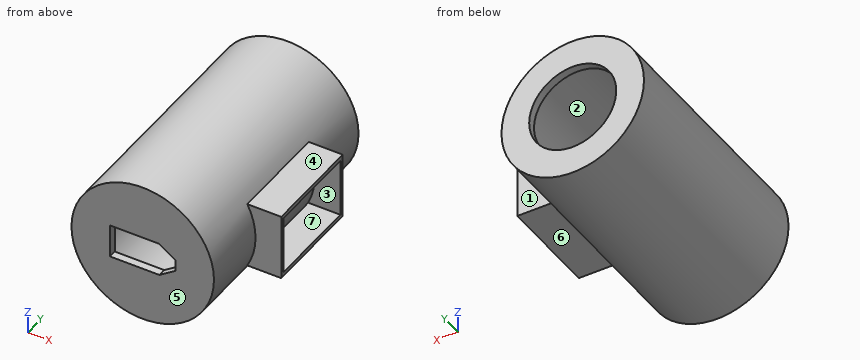
from build123d import *

# Parameters (mm, degrees)
F0_R     = 18
F0_R_2   = 16
F1_DEPTH = 60
F0_R_3   = 11
F2_DEPTH = 8
F3_W     = 25.5
F3_H     = 16.8
F3_W_2   = 23.5
F3_H_2   = 14.8
F4_DEPTH = 24.5
F5_DEPTH = 28.5
F6_DEPTH = 60
F7_DEPTH = 58
F8_DEPTH = 2


with BuildPart() as f1:
    # F0 (on Front) → F1 (new body)
    with BuildSketch(Plane.XZ):
        Circle(F0_R)
        Circle(F0_R_2, mode=Mode.SUBTRACT)
    extrude(amount=F1_DEPTH)

    # F0 (on Front) → F2 (join)
    with BuildSketch(Plane.XZ):
        Circle(F0_R_2)
        Circle(F0_R_3, mode=Mode.SUBTRACT)
    extrude(amount=F2_DEPTH)

    # F3 (on Right) → F4 (join)
    with BuildSketch(Plane.YZ):
        with Locations((-30, 0)):
            Rectangle(F3_W, F3_H)
        with Locations((-30, 0)):
            Rectangle(F3_W_2, F3_H_2, mode=Mode.SUBTRACT)
    extrude(amount=F4_DEPTH)

    # F5 (cut): a face of the model
    f5_faces = [f1.faces().sort_by_distance(p)[0] for p in [
        (7.6317317332, -42.75, 0),
    ]]
    extrude(f5_faces, amount=-F5_DEPTH, mode=Mode.SUBTRACT)

    # F0 (on Front) → F6 (join)
    with BuildSketch(Plane.XZ):
        Circle(F0_R_2)
        Circle(F0_R_3, mode=Mode.SUBTRACT)
        Circle(F0_R_3)
        Polygon((4.2248526588, 4.25), (8.25, 4.25), (8.25, 1.5), (8.25, -1.5), (8.25, -4.25), (4.2248526588, -4.25), (-8.25, -4.25), (-8.25, 4.25), align=None, mode=Mode.SUBTRACT)
        Polygon((8.25, 1.5), (8.25, 4.25), (4.2248526588, 4.25), align=None)
        Polygon((8.25, -4.25), (8.25, -1.5), (4.2248526588, -4.25), align=None)
    extrude(amount=F6_DEPTH)

    # F0 (on Front) → F7 (cut)
    with BuildSketch(Plane.XZ):
        Circle(F0_R_2)
        Circle(F0_R_3, mode=Mode.SUBTRACT)
        Circle(F0_R_3)
        Polygon((4.2248526588, 4.25), (8.25, 4.25), (8.25, 1.5), (8.25, -1.5), (8.25, -4.25), (4.2248526588, -4.25), (-8.25, -4.25), (-8.25, 4.25), align=None, mode=Mode.SUBTRACT)
        Polygon((8.25, 1.5), (8.25, 4.25), (4.2248526588, 4.25), align=None)
        Polygon((8.25, -4.25), (8.25, -1.5), (4.2248526588, -4.25), align=None)
    extrude(amount=F7_DEPTH, mode=Mode.SUBTRACT)

    # F0 (on Front) → F8 (join)
    with BuildSketch(Plane.XZ):
        Circle(F0_R_2)
        Circle(F0_R_3, mode=Mode.SUBTRACT)
    extrude(amount=F8_DEPTH)


solid = f1.part
Check sheet for the modelled part. Datum: model origin and axes. Units: mm. Face numbers are marked on the shaded views. A direction names the side the tool comes from. Give positions to 0.01 mm unless a question says otherwise; leave off trailing zeros. Order: outer loops, then holes, each group sorted by start corner. A loop starts at its lowest first (then second) coordinate and runs counter-clockwise, first axis right, second up. Notation, with made-up numbers: M 83.25,-25 L 120.25,-25 A18 cw 120.25,10 Z; hole C 56.25,35.5 d8. An arc over 180 degrees is marked long. Answer as CSV lines item,"result". Start each with the question number.
Item 1: Thickness scan on line 1 (Y direction, x = 19.5, z = 0); line 2 (Z direction, x = 0, y = -26); line 3 (X direction, y = -15.5, z = -0.5). Record the ranges inside material, lowest first. Write a range as [from, to].
Item 2: Gauge pin test, flat ends, axial feed: P1, Ø2.5, axis at x = 20, y = -28, coming from the -Z side; P2, Ø9, axis at x = 19.5, y = -31, coming from the +Z side; P3, Ø3, axis at x = 18, y = -48, coming from the +Z side; P4, Ø10, axis at y = -14.5, z = -10.5, coming from the +X side. Record the tip position at first contact, or that the pin passes through.
Item 3: Cross-section at B-B on z = 0. Enter the section's corners in (x, y).
Item 4: Cross-section at D-D on z = 13. Enter the section's corners in (x, y), plus the area to 3 significant figures.
Item 5: Tool access check on the marked faces 5, 6 and 7. Record the directions out of +Z, -Z, +X, -X, +Y, -Y that give a thin tool (end or side, any length) a straight path to the whole face; none if there is none.
Item 6: Mould release check, pull along Y, two halves, no side actions. Record for the marked faces 1, 2, 3 and 4: +Y half, -Y half, draft (parallel to the pull), parting line (faces both ways), or undercut.
Item 7: Cross-section at A-A on y = -33.5. Enter the section's corners in (x, z), plus the area to 3 significant figures.
Item 8: Cross-section at C-C on x = 0. Enter the section's corners in (y, z).
Established:
1,line 1,"y = [-42.75, -41.75], [-18.25, -17.25]"
1,line 2,"z = [-18, -16], [16, 18]"
1,line 3,"x = [-17.99, -15.99], [15.99, 17.99]"
2,P1,"stops at z = -8.4"
2,P2,"stops at z = 9.95"
2,P3,"stops at z = 7.19"
2,P4,"stops at x = 24.5"
3,outline,"M -18,-60 L -8.25,-60 L -8.25,-58 L -16,-58 L -16,-2 L -11,-2 L -11,0 L -18,0 Z; M 8.25,-60 L 18,-60 L 18,-42.75 L 24.5,-42.75 L 24.5,-41.75 L 18,-41.75 L 18,-18.25 L 24.5,-18.25 L 24.5,-17.25 L 18,-17.25 L 18,0 L 11,0 L 11,-2 L 16,-2 L 16,-58 L 8.25,-58 Z"
4,outline,"M -12.45,-60 L 12.45,-60 L 12.45,0 L -12.45,0 Z; hole M -9.33,-58 L 9.33,-58 L 9.33,-2 L -9.33,-2 Z"
4,area,"449 mm^2"
5,face 5,"+Z, -Z, +X, -X, -Y"
5,face 6,"-Z, +X, +Y, -Y"
5,face 7,"+X"
6,face 1,"+Y half"
6,face 2,"undercut"
6,face 3,"undercut"
6,face 4,"draft"
7,outline,"M 15.92,-8.4 L 24.5,-8.4 L 24.5,-7.4 L 16.41,-7.4 A18 ccw 16.41,7.4 L 24.5,7.4 L 24.5,8.4 L 15.92,8.4 A18 ccw long Z; hole C 0,0 d32"
7,area,"230 mm^2"
8,outline,"M -60,-18 L 0,-18 L 0,-11 L -2,-11 L -2,-16 L -58,-16 L -58,-4.25 L -60,-4.25 Z; M -60,4.25 L -58,4.25 L -58,16 L -2,16 L -2,11 L 0,11 L 0,18 L -60,18 Z"
